Part print with two shaded views. Sizes in mm from the minimum x, y, z corner. Coordinates: 2 decimals unless noted, no trailing zeros. Write each loop counter-clockwise with the first axis right and the second up, starting at its lowest first coordinate (ties: lowest second). Pieces come first, ordered by that corner, then holes.
Q1. Drill centre lines: probe 1 along X at (y, z) = (8.75, 4.5); probe 2 along X at (y, z) = (7.75, 3.9); probe 3 along Z at (x, y) = (1.5, 1). Where is each one in solid material? Low to high.
Q2. Pin check, flat tips, straight feed: P1, Ø1, axis at y = 4, z = 1.5, coming from the -X side; P2, Ø3, axis at y = 7, z = 4.5, coming from the +X side. Stop position of each tip, or through.
Q3. Band-saw the part on C-C, the plane x = 4.9. Write the cut outline in (y, z).
Q4. Pull direction Z, two halves, no side cores. Call the marked faces 1, 2 and 3: released by +Z, released by -Z, zero draft, split by the parting line, or undercut.
Q5. Band-saw the part on B-B, the plane z = 1.7. Write the cut outline in (x, y) (3 decimals), plus the area to 3 significant figures.
Q6. Band-saw the part on A-A, the plane y = 7. Write the cut outline in (x, z) (1 decimal), plus the area to 3 significant figures.
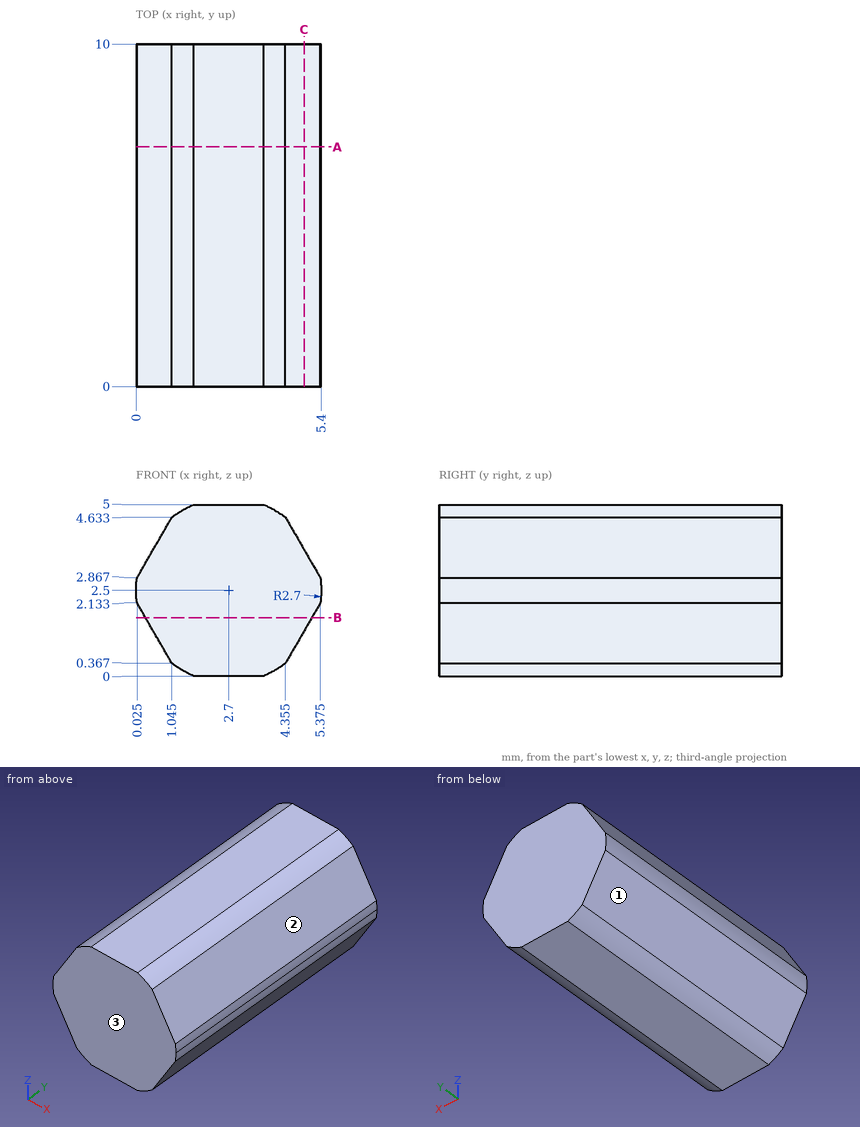
Answer sheet:
1. probe 1: x = 0.97 to 4.43
1. probe 2: x = 0.62 to 4.78
1. probe 3: z = 0.08 to 4.92
2. P1: stops at x = 0.1
2. P2: stops at x = 5.3
3. outline: (0, 1.31) - (10, 1.31) - (10, 3.69) - (0, 3.69) - close
4. face 1: released by -Z
4. face 2: released by +Z
4. face 3: zero draft
5. outline: (0.275, 0) - (5.125, 0) - (5.125, 10) - (0.275, 10) - close
5. area: 48.5 mm2
6. outline: (0, 2.1) - (1, 0.4) arc R2.7 ccw to (1.7, 0) - (3.7, 0) arc R2.7 ccw to (4.4, 0.4) - (5.4, 2.1) arc R2.7 ccw to (5.4, 2.9) - (4.4, 4.6) arc R2.7 ccw to (3.7, 5) - (1.7, 5) arc R2.7 ccw to (1, 4.6) - (0, 2.9) arc R2.7 ccw to start
6. area: 21.3 mm2
